Build history of the part. All positions in model axes, mm. Face numbers are marked on the shaded views. A direction names the side the tool comes from. Round coordinates to 2 decimals unless told otherwise and drop trailing zeros. Write each loop counter-clockwise with the first axis right and the second up, starting at its lowest first coordinate (ties: lowest second). Pieces come first, ordered by that corner, then holes.
from build123d import *

# Parameters (mm, degrees)
BOSS_EXTRUDE1_DEPTH      = 10
BOSS_EXTRUDE1_DEPTH_BACK = 42
SKETCH1_R                = 42.5
SKETCH1_R_2              = 10
SKETCH1_R_3              = 2.55
SKETCH2_R                = 37.5
CUT_EXTRUDE1_DEPTH       = 44
CUT_EXTRUDE2_START       = -42
CUT_EXTRUDE2_DEPTH       = 20
SKETCH4_R                = 14.35
CUT_EXTRUDE3_DEPTH       = 7.9375
CUT_EXTRUDE4_START       = 10
SKETCH5_R                = 4.35
CUT_EXTRUDE4_DEPTH       = 5.5


with BuildPart() as part:
    # Sketch1 → Boss-Extrude1 (new, two sides: drawn at the far end of the back side and taken through both)
    with BuildSketch(Plane(origin=(0, 0, 0), x_dir=(1, 0, 0), z_dir=(0, 1, 0)).offset(-BOSS_EXTRUDE1_DEPTH_BACK)):
        with Locations(Location((0, 0, 0), (0, 0, 270))):
            Circle(SKETCH1_R)
        with Locations(Location((0, 0, 0), (0, 0, 270))):
            Circle(SKETCH1_R_2, mode=Mode.SUBTRACT)
        with Locations(Location((-37.5, 0, 0), (0, 0, 270))):
            Circle(SKETCH1_R_3, mode=Mode.SUBTRACT)
        with Locations(Location((0, -37.5, 0), (0, 0, 270))):
            Circle(SKETCH1_R_3, mode=Mode.SUBTRACT)
        with Locations(Location((37.5, 0, 0), (0, 0, 270))):
            Circle(SKETCH1_R_3, mode=Mode.SUBTRACT)
        with Locations(Location((0, 37.5, 0), (0, 0, 270))):
            Circle(SKETCH1_R_3, mode=Mode.SUBTRACT)
    extrude(amount=BOSS_EXTRUDE1_DEPTH + BOSS_EXTRUDE1_DEPTH_BACK)

    # Sketch2 → Cut-Extrude1 (cut)
    with BuildSketch(Plane(origin=(0, 0, 0), x_dir=(1, 0, 0), z_dir=(0, 1, 0))):
        Circle(SKETCH2_R)
    extrude(amount=-CUT_EXTRUDE1_DEPTH, mode=Mode.SUBTRACT)

    # Sketch3 → Cut-Extrude2 (cut)
    with BuildSketch(Plane(origin=(0, 0, 0), x_dir=(1, 0, 0), z_dir=(0, 1, 0)).offset(CUT_EXTRUDE2_START)):
        Polygon((-37.5, 0), (-37.5, 48.535526989), (-12.5, 48.535526989), (-12.5, 25.15870532), (12.5, 25.15870532), (12.5, 48.535526989), (37.5, 48.535526989), (37.5, 0), align=None)
    extrude(amount=CUT_EXTRUDE2_DEPTH, mode=Mode.SUBTRACT)

    # Sketch4 → Cut-Extrude3 (cut)
    with BuildSketch(Plane(origin=(0, 0, 0), x_dir=(1, 0, 0), z_dir=(0, 1, 0))):
        with Locations(Location((0, 0, 0), (0, 0, 270))):
            Circle(SKETCH4_R)
    extrude(amount=CUT_EXTRUDE3_DEPTH, mode=Mode.SUBTRACT)

    # Sketch5 → Cut-Extrude4 (cut)
    with BuildSketch(Plane(origin=(0, 0, 0), x_dir=(1, 0, 0), z_dir=(0, 1, 0)).offset(CUT_EXTRUDE4_START)):
        with Locations(Location((0, 37.5, 0), (0, 0, 270))):
            Circle(SKETCH5_R)
        with Locations(Location((37.5, 0, 0), (0, 0, 270))):
            Circle(SKETCH5_R)
        with Locations(Location((0, -37.5, 0), (0, 0, 270))):
            Circle(SKETCH5_R)
        with Locations(Location((-37.5, 0, 0), (0, 0, 270))):
            Circle(SKETCH5_R)
    extrude(amount=-CUT_EXTRUDE4_DEPTH, mode=Mode.SUBTRACT)


solid = part.part
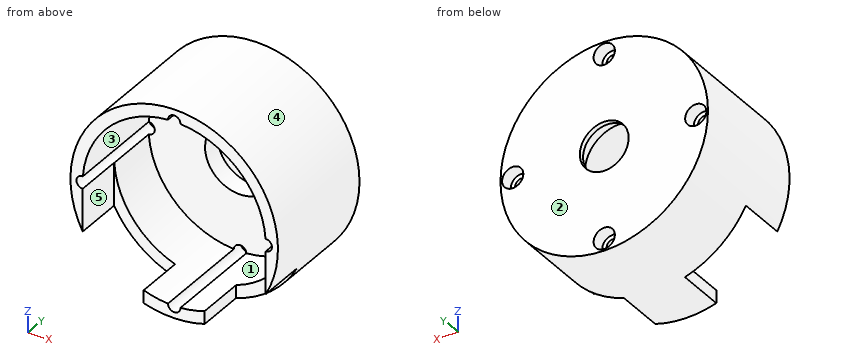
1) Slice it at C-C (z = 0). Write the cut outline in (x, y), plus the area to 3 significant figures.
Results:
outline: (-42.5, -42) - (-40.05, -42) - (-40.05, 4.5) - (-41.85, 4.5) - (-41.85, 10) - (-42.5, 10) - close; (-34.95, 0) - (-14.35, 0) - (-14.35, 7.94) - (-10, 7.94) - (-10, 10) - (-33.15, 10) - (-33.15, 4.5) - (-34.95, 4.5) - close; (10, 7.94) - (14.35, 7.94) - (14.35, 0) - (34.95, 0) - (34.95, 4.5) - (33.15, 4.5) - (33.15, 10) - (10, 10) - close; (40.05, -42) - (42.5, -42) - (42.5, 10) - (41.85, 10) - (41.85, 4.5) - (40.05, 4.5) - close
area: 645 mm2
2) Wall check: L1, parallel to Z at x = 0, y = -30.5; L2, parallel to Y at x = 22.5, z = 24; L3, parallel to Z at x = 12, y = -37.5. Give the ranges that are in metal, low to high.
Results:
L1: z = -42.5 to -40.05, 40.05 to 42.5
L2: y = 0 to 10
L3: z = -40.77 to -35.53, 35.53 to 40.77
3) Which spindle directions (+Z, -Z, +X, -X, +Y, -Y) get a long thin tool onto all of the face, cutting with end or side? Do the marked faces 1 and 2. Say none if no direction does.
Results:
face 1: -Y
face 2: +Z, -Z, +X, -X, +Y
4) Mould opens along Z. For the marked faces 3, 4 and 5 say: released by +Z, released by -Z, zero draft, split by the parting line, or undercut.
Results:
face 3: undercut
face 4: split by the parting line
face 5: zero draft
5) Pin check, flat tips, straight feed: pin 1 Ø6 at (y, z) = (-32, -38.5) entering from -X; pin 2 Ø2.5 at (x, z) = (2, 38.5) entering from +Y; pin 3 Ø1.5 at (y, z) = (-22.5, -4.5) entering from -X. Stop position of each tip, or through.
Results:
pin 1: stops at x = -12.5
pin 2: stops at y = 4.5
pin 3: stops at x = -42.33
6) Slice it at A-A (y = -14.5). Write the cut outline in (x, z), plus the area to 3 significant figures.
Results:
outline: circle Ø85 at (0, 0); hole (-37.41, -2.55) arc R37.5 ccw to (-2.55, -37.41) arc R2.55 ccw (long way) to (2.55, -37.41) arc R37.5 ccw to (37.41, -2.55) arc R2.55 ccw (long way) to (37.41, 2.55) arc R37.5 ccw to (2.55, 37.41) arc R2.55 ccw (long way) to (-2.55, 37.41) arc R37.5 ccw to (-37.41, 2.55) arc R2.55 ccw (long way) to start
area: 1,220 mm2
7) Slice it at B-B (x = 0). Write the cut outline in (y, z).
Results:
outline: (-42, -42.5) - (10, -42.5) - (10, -41.85) - (4.5, -41.85) - (4.5, -40.05) - (-42, -40.05) - close; (-42, 40.05) - (4.5, 40.05) - (4.5, 41.85) - (10, 41.85) - (10, 42.5) - (-42, 42.5) - close; (0, -34.95) - (4.5, -34.95) - (4.5, -33.15) - (10, -33.15) - (10, -10) - (7.94, -10) - (7.94, -14.35) - (0, -14.35) - close; (0, 14.35) - (7.94, 14.35) - (7.94, 10) - (10, 10) - (10, 33.15) - (4.5, 33.15) - (4.5, 34.95) - (0, 34.95) - close
8) Slice it at D-D (y = -27). Write the cut outline in (x, z).
Results:
outline: (-37.5, -20) - (-37.5, -2.55) arc R2.55 cw (long way) to (-37.41, 2.55) arc R37.5 cw to (-2.55, 37.41) arc R2.55 cw (long way) to (2.55, 37.41) arc R37.5 cw to (37.41, 2.55) arc R2.55 cw (long way) to (37.5, -2.55) - (37.5, -20) arc R42.5 ccw (long way) to start; (-12.5, -40.62) arc R42.5 ccw to (12.5, -40.62) - (12.5, -35.36) arc R37.5 cw to (2.55, -37.41) arc R2.55 cw (long way) to (-2.55, -37.41) arc R37.5 cw to (-12.5, -35.36) - close
